Build history of the part. All positions in model axes, mm. A direction names the side the tool comes from. Give positions to 0.01 mm unless a question says otherwise; leave off trailing zeros. Loops run counter-clockwise (first coordinate to the right, second up) from the corner with the lowest first, then second, coordinate; pieces in that order, holes last. Notation, with made-up numbers: M -0.5,16 L 27.5,16 A28 cw 27.5,36 Z; hole C 25,48.25 d3. An arc over 180 degrees is marked long. Put each result on its own line as item: value.
```python
from build123d import *

# Parameters (mm, degrees)
F1_DEPTH = 25.4
F2_DEPTH = 25.4
F3_DEPTH = 25.4


with BuildPart() as f1:
    # F0 (on Front) → F1 (new body)
    with BuildSketch(Plane.XZ):
        Polygon((-23.7604218155, 67.1883597866), (-74.5604218155, 67.1883597866), (-74.5604218155, 41.7883597866), (-49.1604218155, 41.7883597866), (-49.1604218155, -34.4116402134), (27.0395781845, -34.4116402134), (27.0395781845, -9.0116402134), (-23.7604218155, -9.0116402134), align=None)
    extrude(amount=F1_DEPTH)

    # F2 (add): a face of the model
    f2_faces = [f1.faces().sort_by_distance(p)[0] for p in [
        (-29.2032789584, -25.4, 10.9455026437),
    ]]
    extrude(f2_faces, amount=F2_DEPTH)

    # F3 (add): a face of the model
    f3_faces = [f1.faces().sort_by_distance(p)[0] for p in [
        (-29.2032789584, -50.8, 10.9455026437),
    ]]
    extrude(f3_faces, amount=F3_DEPTH)


solid = f1.part
```
Q1. Drop flat-ended pins along their axis: pin 1 Ø1 at (y, z) = (-51.5, 36) entering from +X; pin 2 Ø3 at (x, y) = (8, -56.5) entering from +Z; pin 3 Ø12 at (y, z) = (-22.5, -4) entering from -X. Give the stop position or say it passes through.
Here are the results:
pin 1: x = -23.76
pin 2: z = -9.01
pin 3: x = -49.16
Q2. Slice it at C-C (z = 45). List the corners of the cut face in (x, y), and give its area (3 significant figures).
Here are the results:
outline: M -74.56,-76.2 L -23.76,-76.2 L -23.76,0 L -74.56,0 Z
area: 3,870 mm²
Q3. Probe line 1 (X direction, y = -58, z = 45); line 2 (Z direction, x = -9, y = -13.5); line 3 (X direction, y = -52.5, z = 18.5). List the from-to ranges inside material, lowest first. Write a range as from..to.
Here are the results:
line 1: -74.56..-23.76
line 2: -34.41..-9.01
line 3: -49.16..-23.76
Q4. Slice it at B-B (x = -14). List the corners of the cut face in (y, z), and give its area (3 significant figures).
Here are the results:
outline: M -76.2,-34.41 L 0,-34.41 L 0,-9.01 L -76.2,-9.01 Z
area: 1,940 mm²
Q5. Slice it at A-A (y = -67.5). List the corners of the cut face in (x, z), and give its area (3 significant figures).
Here are the results:
outline: M -74.56,41.79 L -49.16,41.79 L -49.16,-34.41 L 27.04,-34.41 L 27.04,-9.01 L -23.76,-9.01 L -23.76,67.19 L -74.56,67.19 Z
area: 4,520 mm²
Q6. Tool access for faces 1 (the flat face through (-36, -76.2, 17)), 2 (the flat face through (2, -38, -9.012)), 3 (the flat face through (-49.16, -38, 4)): list every direction of +Z, -Z, +X, -X, +Y, -Y with a clear straight run to the whole face (end or side of a thin tool).
Here are the results:
face 1: +Z, -Z, +X, -X, -Y
face 2: +Z, +X, +Y, -Y
face 3: -Z, -X, +Y, -Y
